```python
from build123d import *

# Parameters (mm, degrees)
BOSS_EXTRUDE1_DEPTH = 10.795
BOSS_EXTRUDE2_DEPTH = 3.175
CUT_EXTRUDE1_DEPTH  = 55.133861737
CUT_EXTRUDE3_DEPTH  = 50.9999
SKETCH5_R           = 1.524
CUT_EXTRUDE4_DEPTH  = 14.97


with BuildPart() as part:
    # Sketch1 → Boss-Extrude1 (new body)
    with BuildSketch(Plane(origin=(0, 0, 0), x_dir=(1, 0, 0), z_dir=(0, 1, 0))):
        with BuildLine():
            Line((0, 0), (33.655, 0))
            Line((33.655, 0), (33.655, -7.62))
            Line((33.655, -7.62), (45.882312708, -36.965550498))
            ThreePointArc((45.882312708, -36.965550498), (45.852364547, -37.905157075), (45.166785817, -38.548382711))
            Line((45.166785817, -38.548382711), (30.715714183, -44.001617289))
            ThreePointArc((30.715714183, -44.001617289), (29.6938714, -44.069401845), (28.806656699, -43.557926045))
            ThreePointArc((28.806656699, -43.557926045), (24.828111607, -40.263477877), (20.0025, -38.420740133))
            Line((20.0025, -38.420740133), (20.0025, -38.1))
            Line((20.0025, -38.1), (20.0025, -34.29))
            Line((20.0025, -34.29), (13.6525, -34.29))
            Line((13.6525, -34.29), (13.6525, -38.1))
            Line((13.6525, -38.1), (13.6525, -38.420740133))
            ThreePointArc((13.6525, -38.420740133), (8.826888393, -40.263477877), (4.848343301, -43.557926045))
            ThreePointArc((4.848343301, -43.557926045), (3.9611286, -44.069401845), (2.939285817, -44.001617289))
            Line((2.939285817, -44.001617289), (-11.511785817, -38.548382711))
            ThreePointArc((-11.511785817, -38.548382711), (-12.197364547, -37.905157075), (-12.227312708, -36.965550498))
            Line((-12.227312708, -36.965550498), (0, -7.62))
            Line((0, -7.62), (0, 0))
        make_face()
    extrude(amount=BOSS_EXTRUDE1_DEPTH)

    # Sketch2 → Boss-Extrude2 (add)
    with BuildSketch(Plane.XZ):
        Polygon((16.8275, 0), (-8.17245, 0), (-8.17245, 49.9999), (41.82745, 49.9999), (41.82745, 0), align=None)
    extrude(amount=BOSS_EXTRUDE2_DEPTH)

    # Sketch3 → Cut-Extrude1 (cut, through all)
    with BuildSketch(Plane.ZY.offset(8.17245)):
        Polygon((7.62, -3.175), (0, 0), (0, -3.175), align=None)
    extrude(amount=-CUT_EXTRUDE1_DEPTH, mode=Mode.SUBTRACT)

    # Sketch4 → Cut-Extrude3 (cut, through all)
    with BuildSketch(Plane(origin=(0, 0, 0), x_dir=(-1, 0, 0), z_dir=(0, 0, -1))):
        Polygon((-41.82745, 0), (-47.971594171, 0), (-47.971594171, 6.144144171), align=None)
        Polygon((8.17245, 0), (16.073165013, 0), (16.073165013, 7.900715013), align=None)
    extrude(amount=-CUT_EXTRUDE3_DEPTH, mode=Mode.SUBTRACT)

    # Sketch5 → Cut-Extrude4 (cut, through all)
    with BuildSketch(Plane.XZ.offset(3.175)):
        with Locations((6.8274946, 34.9999554)):
            Circle(SKETCH5_R)
        with Locations((26.8275054, 34.9999554)):
            Circle(SKETCH5_R)
        with Locations((6.8274946, 14.9999446)):
            Circle(SKETCH5_R)
        with Locations((26.8275054, 14.9999446)):
            Circle(SKETCH5_R)
    extrude(amount=-CUT_EXTRUDE4_DEPTH, mode=Mode.SUBTRACT)


solid = part.part
```
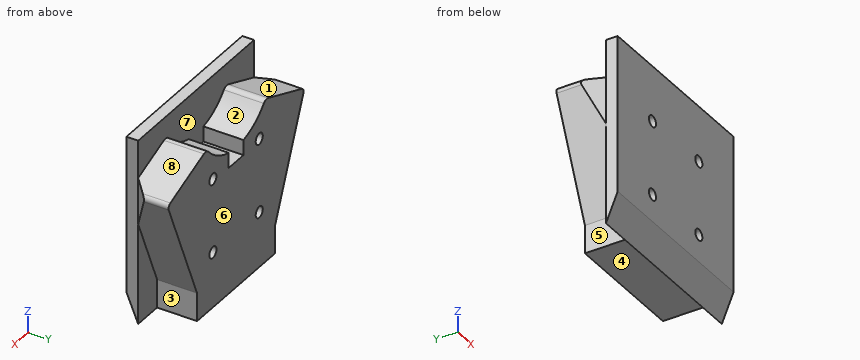
Model file for the job. Use its own axes, mm. Face numbers are marked on the shaded views. A direction names the side the tool comes from. Give positions to 0.01 mm unless a question says otherwise; leave off trailing zeros. Loops run counter-clockwise (first coordinate to the right, second up) from the corner with the lowest first, then second, coordinate; pieces in that order, holes last. Notation, with made-up numbers: (-15.5, 36) -> (9.5, 36) arc R17 cw to (9.5, 62) -> close; hole circle Ø8 at (65.5, -24). An arc over 180 degrees is marked (long way). Write each question's results on one line, items separated by ' | '.
(1) Pull direction X, two halves, no side cores. Call the marked faces 6, 7 and 8: released by +X, released by -X, zero draft, split by the parting line, or undercut.
Geometry results:
face 6: zero draft | face 7: undercut | face 8: released by +X
(2) Probe line 1 along Z through (x, y) = (8, 5.5); line 2 along X through (y, z) = (9.25, 16); line 3 along Z through (x, y) = (16.5, 7). List the from-to ranges inside material, lowest first.
Geometry results:
line 1: z = 0 to 14.03, 15.97 to 34.03, 35.97 to 40.78 | line 2: x = -3.49 to 5.68, 7.98 to 25.68, 27.98 to 37.15 | line 3: z = 0 to 34.29
(3) Flat gauge pins, fed straight in: pin 1 Ø4 at (y, z) = (7, 5) entering from +X (3 decimals); pin 2 Ø2.5 at (y, z) = (-1, 28) entering from -X; pin 3 Ø1.8 at (x, z) = (26.83, 15) entering from -Y; pin 4 Ø4.5 at (x, z) = (22.5, 44) entering from +Y. Where does each tip first touch, or does it go through?
Geometry results:
pin 1: stops at x = 33.655 | pin 2: stops at x = -8.42 | pin 3: passes through | pin 4: stops at y = 0
(4) Cut at B-B on z = 19. List the corners of the cut face in (x, y) (3 decimals), and give its area (3 significant figures).
Geometry results:
outline: (-8.172, -3.175) -> (41.827, -3.175) -> (41.827, 0) -> (38.397, 0) -> (38.397, 10.795) -> (-4.742, 10.795) -> (-4.742, 0) -> (-8.172, 0) -> close | area: 624 mm²
(5) Tool access for the marked faces 1, 2, 3, 4 and 5: list every direction of +Z, -Z, +X, -X, +Y, -Y with a clear straight run to the whole face (end or side of a thin tool).
Geometry results:
face 1: +Z, -X, +Y | face 2: +Z, +Y | face 3: -Z, +X, +Y | face 4: -Z, +X, -X, +Y, -Y | face 5: -Z, -X, +Y
(6) Cut at A-A on y = 2. Give the number of separate pieces and of enclosed holes in the cut face, and give its area (3 significant figures).
Geometry results:
separate pieces: 1 | enclosed holes: 4 | area: 1,750 mm²
(7) Cut at C-C on x = 22.5. List the corners of the cut face in (y, z) (3 decimals).
Geometry results:
outline: (-3.175, 7.62) -> (0, 0) -> (10.795, 0) -> (10.795, 39.148) -> (0, 39.148) -> (0, 50) -> (-3.175, 50) -> close
(8) Cut at D-D on z = 10.5. List the corners of the cut face in (x, y) (3 decimals).
Geometry results:
outline: (-8.172, -3.175) -> (41.827, -3.175) -> (41.827, 0) -> (34.855, 0) -> (34.855, 10.795) -> (-1.2, 10.795) -> (-1.2, 0) -> (-8.172, 0) -> close
